from build123d import *

# Parameters (mm, degrees)
BOSS_EXTRUDE1_DEPTH = 50
SKETCH2_R           = 1.6
CUT_EXTRUDE1_DEPTH  = 10


with BuildPart() as part:
    # Sketch1 → Boss-Extrude1 (new body)
    with BuildSketch(Plane.XY):
        with BuildLine():
            Line((55, 0), (50, 0))
            ThreePointArc((50, 0), (0, 50), (-50, 0))
            Line((-50, 0), (-55, 0))
            ThreePointArc((-55, 0), (0, 55), (55, 0))
        make_face()
    extrude(amount=BOSS_EXTRUDE1_DEPTH)

    # Sketch2 → Cut-Extrude1 (cut)
    with BuildSketch(Plane(origin=(0, 0, 0), x_dir=(-1, 0, 0), z_dir=(0, 0, -1))):
        with Locations((0, 52.5)):
            Circle(SKETCH2_R)
        with Locations((33.746349509, 40.217333264)):
            Circle(SKETCH2_R)
        with Locations((51.702407033, 9.116529328)):
            Circle(SKETCH2_R)
        with Locations((-51.702407033, 9.116529328)):
            Circle(SKETCH2_R)
        with Locations((-33.746349509, 40.217333264)):
            Circle(SKETCH2_R)
    extrude(amount=-CUT_EXTRUDE1_DEPTH, mode=Mode.SUBTRACT)


solid = part.part
Input: part model. Units: mm. Frame: model coordinates. A direction names the side the tool comes from. Round coordinates to 2 decimals unless told otherwise and drop trailing zeros. Order: outer loops, then holes, each group sorted by start corner. A loop starts at its lowest first (then second) coordinate and runs counter-clockwise, first axis right, second up.
1. Pin query (flat end, axial travel): P1, Ø12, axis at x = 40, z = 7, coming from the -Y side; P2, Ø1.5, axis at x = -21.5, z = 24, coming from the +Y side; P3, Ø3, axis at x = -51.7, y = 9.12, coming from the -Z side. Return the tip coordinate at first contact, or that it passes through.
The answers:
P1: stops at y = 19.6
P2: stops at y = 50.94
P3: stops at z = 10
2. Cut plane C-C, the plane y = 52.5. Output: boundary loops of the cut face in (x, z).
The answers:
outline: (-16.39, 0) - (-1.6, 0) - (-1.6, 10) - (1.6, 10) - (1.6, 0) - (16.39, 0) - (16.39, 50) - (-16.39, 50) - close
3. Cut plane B-B, the plane y = 15.5. Output: boundary loops of the cut face in (x, z).
The answers:
outline: (-52.77, 0) - (-47.54, 0) - (-47.54, 50) - (-52.77, 50) - close; (47.54, 0) - (52.77, 0) - (52.77, 50) - (47.54, 50) - close
4. Set-up query: faces 1 (the face through (-34.485, 38.798, 4.93)), 2 (the face through (4, 50, 50)). Return all of +Z, -Z, +X, -X, +Y, -Y with unobstructed straight access to the full face (end or side cutting, diameter ignored); none if empty.
The answers:
face 1: -Z
face 2: +Z, +X, -X, +Y, -Y
5. Material intervals for line 1 (Y direction, x = 0, z = 6.75); line 2 (X direction, y = 9.5, z = 5); line 3 (X direction, y = 19.5, z = 44.5), sorted ascending.
The answers:
line 1: y = 50 to 50.9, 54.1 to 55
line 2: x = -54.17 to -53.26, -50.15 to -49.09, 49.09 to 50.15, 53.26 to 54.17
line 3: x = -51.43 to -46.04, 46.04 to 51.43
6. Cut plane A-A, the plane x = 0. Output: boundary loops of the cut face in (y, z).
The answers:
outline: (50, 0) - (50.9, 0) - (50.9, 10) - (54.1, 10) - (54.1, 0) - (55, 0) - (55, 50) - (50, 50) - close
7. Mould query, pull axis X, two halves, no side actions, for faces 3 (the face through (-0.86, 53.85, 4.93)), 4 (the face through (-1.209, 54.987, 24.65)), 5 (the face through (53, 0, 25)). Classes: released by +X, released by -X, zero draft, split by the parting line, or undercut.
The answers:
face 3: undercut
face 4: split by the parting line
face 5: zero draft
8. Cut plane D-D, the plane z = 20. Output: boundary loops of the cut face in (x, y), then the cut area to 3 significant figures.
The answers:
outline: (-55, 0) - (-50, 0) arc R50 cw to (50, 0) - (55, 0) arc R55 ccw to start
area: 825 mm2
